from build123d import *

# Parameters (mm, degrees)
SKETCH_1_W                   = 60
SKETCH_1_H                   = 55
EXTRUDE_1_DEPTH              = 6
HOLE_WIZARD_M4_1_D           = 2.9
HOLE_WIZARD_M4_1_DEPTH       = 10
SKETCH_5_R                   = 20
CUT_EXTRUDE_1_DEPTH          = 7
SKETCH_6_W                   = 60
SKETCH_6_H                   = 55
CUT_EXTRUDE_2_DEPTH          = 7
EXTRUDE_2_DEPTH              = 6
EXTRUDE_3_DEPTH              = 6
EXTRUDE_4_DEPTH              = 4
CUT_EXTRUDE_3_DEPTH          = 11
CUT_EXTRUDE_4_DEPTH          = 6
FILLET_1_R                   = 2
EXTRUDE_5_DEPTH              = 6
CHAMFER_2_SIZE               = 5
FILLET_4_R                   = 2
CHAMFER_3_SIZE               = 1
HOLE_WIZARD_M3_2_D           = 3.3
HOLE_WIZARD_M3_2_DEPTH       = 10
HOLE_WIZARD_M3_2_CBORE_D     = 6.5
HOLE_WIZARD_M3_2_CBORE_DEPTH = 3.4
HOLE_WIZARD_M3_2_TIP         = 0.991420021


with BuildPart() as part:
    # ｽｹｯﾁ1 → ﾎﾞｽ - 押し出し1 (new body)
    with BuildSketch(Plane.XY):
        Rectangle(SKETCH_1_W, SKETCH_1_H)
    extrude(amount=EXTRUDE_1_DEPTH)

    # M4 すきま穴1
    with Locations(Plane.XY.offset(6)):
        with Locations((-20, -18), (23, 20)):
            Hole(HOLE_WIZARD_M4_1_D / 2, depth=HOLE_WIZARD_M4_1_DEPTH)

    # ｽｹｯﾁ5 → ｶｯﾄ - 押し出し1 (cut, through all)
    with BuildSketch(Plane.XY.offset(6)):
        Circle(SKETCH_5_R)
    extrude(amount=-CUT_EXTRUDE_1_DEPTH, mode=Mode.SUBTRACT)

    # ｽｹｯﾁ6 → ｶｯﾄ - 押し出し2 (cut, through all)
    with BuildSketch(Plane.XY.offset(6)):
        Rectangle(SKETCH_6_W, SKETCH_6_H)
        with BuildLine():
            ThreePointArc((-17.351208814, -20.997316342), (-22.997316342, -20.648791186), (-22.648791186, -15.002683658))
            Line((-22.648791186, -15.002683658), (-21.007829355, -13.552531342))
            ThreePointArc((-21.007829355, -13.552531342), (-16.554944912, 18.733227137), (16.03335661, 19.181539975))
            Line((16.03335661, 19.181539975), (20.351208814, 22.997316342))
            ThreePointArc((20.351208814, 22.997316342), (25.997316342, 22.648791186), (25.648791186, 17.002683658))
            Line((25.648791186, 17.002683658), (21.271672672, 13.134532414))
            ThreePointArc((21.271672672, 13.134532414), (24.04986296, 6.826718948), (25, 0))
            ThreePointArc((25, 0), (10.810307191, -22.541900062), (-15.650980674, -19.494789148))
            Line((-15.650980674, -19.494789148), (-17.351208814, -20.997316342))
        make_face(mode=Mode.SUBTRACT)
    extrude(amount=-CUT_EXTRUDE_2_DEPTH, mode=Mode.SUBTRACT)

    # ｽｹｯﾁ7 → ﾎﾞｽ - 押し出し2 (add)
    with BuildSketch(Plane.XY.offset(6)):
        with BuildLine():
            Line((0, 25), (-21.5, 25))
            Line((-21.5, 25), (-21.5, 12.757350822))
            ThreePointArc((-21.5, 12.757350822), (-12.370655388, 21.724798855), (0, 25))
        make_face()
        with BuildLine():
            ThreePointArc((-17.351208814, -20.997316342), (-18.583890076, -21.74094008), (-20, -22))
            Line((-20, -22), (-11.874342087, -22))
            ThreePointArc((-11.874342087, -22), (-13.819546614, -20.833149819), (-15.650980674, -19.494789148))
            Line((-15.650980674, -19.494789148), (-17.351208814, -20.997316342))
        make_face()
        with BuildLine():
            ThreePointArc((-21.007829355, -13.552531342), (-21.25763315, -13.157242601), (-21.5, -12.757350822))
            Line((-21.5, -12.757350822), (-21.5, -13.987472843))
            Line((-21.5, -13.987472843), (-21.007829355, -13.552531342))
        make_face()
    extrude(amount=-EXTRUDE_2_DEPTH)

    # ｽｹｯﾁ8 → ﾎﾞｽ - 押し出し3 (add)
    with BuildSketch(Plane.XY.offset(6)):
        with BuildLine():
            Line((-21.5, 12.757350822), (-21.5, 25))
            Line((-21.5, 25), (-45.078427125, 1.421572875))
            Line((-45.078427125, 1.421572875), (-22.82842714, -20.828427109))
            ThreePointArc((-22.82842714, -20.828427109), (-23.998099778, -17.876719173), (-22.648791186, -15.002683658))
            Line((-22.648791186, -15.002683658), (-21.5, -13.987472843))
            Line((-21.5, -13.987472843), (-21.5, -12.757350822))
            ThreePointArc((-21.5, -12.757350822), (-25, 0), (-21.5, 12.757350822))
        make_face()
    extrude(amount=-EXTRUDE_3_DEPTH)

    # ｽｹｯﾁ9 → ﾎﾞｽ - 押し出し4 (add)
    with BuildSketch(Plane(origin=(0, 0, 0), x_dir=(-1, 0, 0), z_dir=(0, 0, -1))):
        Polygon((25.279437252, -4.235281374), (32.350505063, -11.306349186), (45.078427125, 1.421572875), (38.007359313, 8.492640687), align=None)
    extrude(amount=EXTRUDE_4_DEPTH)

    # ｽｹｯﾁ10 → ｶｯﾄ - 押し出し3 (cut, through all)
    with BuildSketch(Plane(origin=(0, 0, -4), x_dir=(-1, 0, 0), z_dir=(0, 0, -1))):
        Polygon((38.007359313, 8.492640687), (21.5, 25), (10.186291501, 25), (39.421572875, -4.235281374), (45.078427125, 1.421572875), align=None)
    extrude(amount=-CUT_EXTRUDE_3_DEPTH, mode=Mode.SUBTRACT)

    # ｽｹｯﾁ12 → ｶｯﾄ - 押し出し4 (cut)
    with BuildSketch(Plane.XY.offset(6)):
        Polygon((-39.421572875, -4.235281374), (-25.656854249, -18), (-21.414213562, -13.757359313), (-35.178932188, 0.007359313), align=None)
    extrude(amount=-CUT_EXTRUDE_4_DEPTH, mode=Mode.SUBTRACT)

    # ﾌｨﾚｯﾄ1
    fillet_1_edges = [part.edges().sort_by_distance(p)[0] for p in [
        (-25.279437252, -4.235281374, -2),
        (-32.350505063, 2.835786438, -2),
        (-25.656854249, -18, 3),
    ]]
    fillet(fillet_1_edges, radius=FILLET_1_R)

    # ｽｹｯﾁ13 → ﾎﾞｽ - 押し出し5 (add)
    with BuildSketch(Plane.XY):
        Polygon((-32.350505063, -11.306349186), (-28.107864376, -7.063708499), (-35.178932188, 0.007359313), (-39.421572875, -4.235281374), align=None)
    extrude(amount=EXTRUDE_5_DEPTH)

    # 面取り2
    chamfer_2_edges = [part.edges().sort_by_distance(p)[0] for p in [
        (-35.886038969, -7.77081528, 6),
    ]]
    chamfer(chamfer_2_edges, length=CHAMFER_2_SIZE)

    # ﾌｨﾚｯﾄ4
    fillet_4_edges = [part.edges().sort_by_distance(p)[0] for p in [
        (-10.186291501, 25, 3),
        (-21.414213562, -13.757359313, 3),
        (-32.350505063, -4.235281374, 6),
        (-35.886038969, -7.77081528, 1),
        (21.271672672, 13.134532414, 3),
        (16.03335661, 19.181539975, 3),
        (-11.874342087, -22, 3),
    ]]
    fillet(fillet_4_edges, radius=FILLET_4_R)

    # 面取り3
    chamfer_3_edges = [part.edges().sort_by_distance(p)[0] for p in [
        (-21.53073374, -21.695518126, 6),
        (-21.53073374, -21.695518126, 0),
        (-23.535533914, -20.121320336, 0),
        (-29.522077939, -8.477922061, -4),
        (-32.350505063, -11.306349186, -1.914213562),
        (-35.886038969, -7.77081528, -4),
        (-36.593145751, -1.406854249, -4),
        (-28.814971157, -0.699747468, -4),
        (-32.350505063, 2.007359313, -4),
        (-26.107864376, -4.235281374, -4),
        (-23.535533906, -15.878679656, 6),
        (-23.535533906, -15.878679656, 0),
        (-23.535533914, -20.121320336, 6),
        (-24.828427125, -18, 6),
        (-24.828427125, -18, 0),
        (24.071292776, 15.608615296, 6),
        (24.071292776, 15.608615296, 0),
        (17.805324329, -17.549086174, 0),
        (17.805324329, -17.549086174, 6),
        (7.771710455, 23.761323966, 6),
        (7.771710455, 23.761323966, 0),
        (18.815379015, 21.640071403, 6),
        (18.815379015, 21.640071403, 0),
        (-39.421572875, -4.235281374, -1.914213562),
        (-37.653805922, -2.467514421, 3.5),
        (-23.036165235, 12.150126266, 6),
        (-22.268398282, 12.917893219, 0),
        (-35.841448632, -0.655157131, 5.847759065),
        (-39.313922278, -4.127630777, 0.93693974),
        (-25.468145751, -9.703427125, 0),
        (-4.678932188, 25, 0),
        (-16.184658438, -22, 0),
        (-10.123231241, 24.847759065, 0),
        (-28.168524548, -7.124368671, 6),
        (-25.468145751, -9.703427125, 6),
        (-10.123231241, 24.847759065, 6),
        (-30.58273811, -9.538582233, 3.5),
        (-28.77038082, -7.726224943, 5.847759065),
        (-32.242854466, -11.198698589, 0.93693974),
        (21.8499093, 13.07067214, 0),
        (21.8499093, 13.07067214, 6),
        (16.046656493, 19.783578925, 0),
        (16.046656493, 19.783578925, 6),
        (-11.897912356, -22.056349368, 6),
        (-11.897912356, -22.056349368, 0),
        (-22.242640687, -13.757359313, 6),
        (-22.242640687, -13.757359313, 0),
        (-20, 0, 0),
        (-20, 0, 6),
        (25.997316342, 22.648791186, 0),
        (25.997316342, 22.648791186, 6),
        (-16.184658438, -22, 6),
        (-4.678932188, 25, 6),
    ]]
    chamfer(chamfer_3_edges, length=CHAMFER_3_SIZE)

    # M3 六角穴付き頭ねじ用座ぐり穴2
    with Locations(Plane.XY.offset(6)):
        with Locations((-32.350505063, -4.235281374)):
            CounterBoreHole(HOLE_WIZARD_M3_2_D / 2, HOLE_WIZARD_M3_2_CBORE_D / 2, HOLE_WIZARD_M3_2_CBORE_DEPTH, depth=HOLE_WIZARD_M3_2_DEPTH)
            with Locations((0, 0, -(HOLE_WIZARD_M3_2_DEPTH + HOLE_WIZARD_M3_2_TIP / 2))):  # 118° drill point
                Cone(0, HOLE_WIZARD_M3_2_D / 2, HOLE_WIZARD_M3_2_TIP, mode=Mode.SUBTRACT)


solid = part.part
Work out the finished part from the listing and answer in its coordinate system (mm). A direction names the side the tool comes from. Give positions to 0.01 mm unless a question says otherwise; leave off trailing zeros. Loops run counter-clockwise (first coordinate to the right, second up) from the corner with the lowest first, then second, coordinate; pieces in that order, holes last. Notation, with made-up numbers: (3, -6) - (21, -6) arc R21 cw to (21, 3) - close; hole circle Ø1 at (78, -2.75). An arc over 180 degrees is marked (long way). Answer in a Markdown table with one row per item. Add a question column.
Q1. Determine the mould class of faces 1 (the flat face through (-16, -22, 3)), 2 (the conical face through (-9.9, 24.4, 5.5)), 3 (the conical face through (25.33, 22.15, 5.83)) for opening direction X: released by +X, released by -X, zero draft, split by the parting line, or undercut.
Q2. The part is cut by section A-A (z = -1.25). Determine the outline of the cut face in (x, y).
Q3. Each of these flat-tipped pins is pushed along its axis until it touches: P1, Ø6, axis at x = 5, y = -17.5, coming from the +Z side; P2, Ø3, axis at x = -32.5, y = -3, coming from the +Z side; P3, Ø2, axis at x = 17, y = 10, coming from the +Z side; P4, Ø1, axis at x = -29.5, z = 4.5, coming from the -Y side. Where does it stop, or does it pass through?
Q4. The part is cut by section B-B (z = 4). Determine the outline of the cut face in (x, y), and give its area (3 significant figures).
Q5. A tool of negligible diameter and unlimited length cuts with its end or side. For faces 4 (the flat face through (19.16, 21.29, 0.51)), 5 (the flat face through (23.723, 15.959, 0.507)), 6 (the flat face through (-34, -3, 2.6)), 7 (the flat face through (-27.652, 7.534, 1.833)), 8 (the cylindrical face through (-24.83, -18.02, 2.97)), from which of +Z, -Z, +X, -X, +Y, -Y can it reach the whole face along a straight path? Write none if from no direction.
Q6. Consider line 1 along X through (y, z) = (-17.5, 1.25); line 2 along X through (y, z) = (-3.5, 4); line 3 along Y through (x, z) = (0, 2.8). Determine where each line is inside the solid, lowest interval first.
Solution:
| question | item | result |
|---|---|---|
| 1 | face 1 | zero draft |
| 1 | face 2 | released by -X |
| 1 | face 3 | undercut |
| 2 | outline | (-38.71, -4.94) - (-33.06, -10.6) - (-31.64, -10.6) - (-26.69, -5.65) arc R2 ccw to (-26.69, -2.82) - (-30.94, 1.42) arc R2 ccw to (-33.76, 1.42) - (-38.71, -3.53) - close; hole circle Ø3.3 at (-32.35, -4.24) |
| 3 | P1 | stops at z = 6 |
| 3 | P2 | stops at z = 2.6 |
| 3 | P3 | stops at z = 5.72 |
| 3 | P4 | stops at y = -8.24 |
| 4 | outline | (-36.59, -2.82) - (-35.58, -3.84) arc R3.25 cw (long way) to (-31.95, -7.46) - (-30.94, -8.48) - (-29.23, -8.19) - (-28.11, -7.06) - (-22.83, -12.34) arc R2 cw to (-22.83, -15.17) - (-24.24, -16.59) arc R2 ccw to (-24.24, -19.41) - (-22.83, -20.83) arc R4 ccw to (-20, -22) - (-12.37, -22) arc R2 cw to (-11.45, -22.22) arc R25 ccw to (22.05, 11.77) arc R2 cw to (22.49, 14.21) - (25.65, 17) arc R4 ccw to (20.35, 23) - (17.28, 20.28) arc R2 cw to (14.77, 20.17) arc R25 ccw to (0, 25) - (-9.36, 25) arc R2 ccw to (-10.77, 24.41) - (-36.3, -1.11) - close; hole circle Ø2.9 at (-20, -18); hole circle Ø40 at (0, 0); hole circle Ø2.9 at (23, 20) |
| 4 | area | 957 mm² |
| 5 | face 4 | -Z, +Y |
| 5 | face 5 | -Z, +X |
| 5 | face 6 | +Z |
| 5 | face 7 | +Z, -Z, -X, +Y |
| 5 | face 8 | +Z, -Z, -X |
| 6 | line 1 | x = -24.76 to -21.36, -18.64 to -9.68, 9.68 to 17.85 |
| 6 | line 2 | x = -35.91 to -35.52, -29.18 to -19.69, 19.69 to 24.75 |
| 6 | line 3 | y = -25 to -20, 20 to 25 |
